Autodesk Inventor part; units mm, degrees
ref_plane "YZ Plane" through (0, 0, 0) normal (1, 0, 0) x (0, 1, 0)
ref_plane "XZ Plane" through (0, 0, 0) normal (0, 1, 0) x (-1, 0, 0)
ref_plane "XY Plane" through (0, 0, 0) normal (0, 0, 1) x (1, 0, 0)
sketch "Эскиз1" plane through (0, 0, 0) normal (0, 1, 0) x (-1, 0, 0)
  arc A0 (42, 49.6085) -> (42, -49.6085) centre (0, 0) ccw
  line L0 (42, 49.6085) -> (42, -49.6085)
  arc A1 (42, -49.6085) -> (42, 49.6085) centre (0, 0) ccw construction
  line L1 (34, 55.3986) -> (34, -55.3986) construction
  circle A2 centre (34, 45) radius 1.5
  circle A3 centre (34, -45) radius 1.5
  line L2 (-28, 58.66) -> (-28, -58.66) construction
  line L3 (0, 0) -> (-28, -55) construction
  line L4 (0, 0) -> (-56.516, 0) construction
  circle A4 centre (-56.516, 0) radius 2
  circle A5 centre (-28, 45) radius 1.5
  circle A6 centre (-28, -45) radius 1.5
  dimension "d0" = 130
  dimension "d1" = 42
  dimension "d4" = 8
  dimension "d5" = 3
  dimension "d6" = 3
  dimension "d7" = 45
  dimension "d8" = 45
  dimension "d9" = 70
  dimension "d12" = 55
  dimension "d16" = 61.7171
  dimension "d18" = 4
  dimension "d20" = 3
  dimension "d21" = 45
  dimension "d22" = 3
  dimension "d38" = 56.516
extrude "Выдавливание1" add sketch "Эскиз1" along normal blind 3
sketch "Эскиз2" plane through (0, 3, 0) normal (0, 1, 0) x (1, 0, 0)
  circle A0 centre (-34, -45) radius 1.5
  circle A1 centre (-34, 45) radius 1.5
  line L0 (-34, -45) -> (-34, 45) construction
  circle A2 centre (0, 0) radius 55 construction
  line L1 (0, 0) -> (0, -55) construction
  line L2 (0, 0) -> (45.0534, -31.5467) construction
  circle A3 centre (45.0534, -31.5467) radius 1.5
  circle A4 centre (56.516, 0) radius 2
  line L3 (0, 0) -> (56.516, 0) construction
  circle A5 centre (45.0534, 31.5467) radius 1.5
  circle A6 centre (-34, -32) radius 1.5
  circle A7 centre (-34, 32) radius 1.5
  line L4 (-42, 49.6085) -> (-42, -49.6085)
  point P0 (-42, 0)
  point P1 (-34, 0)
  dimension "d25" = 110
  dimension "d26" = 55
  dimension "d28" = 3
  dimension "d34" = 3
  dimension "d35" = 3
  dimension "d36" = 32
  dimension "d37" = 32
extrude "Выдавливание2" cut sketch "Эскиз2" against normal blind 10 contours A3 | A5 | A6 | A7
chamfer "Фаска1" distance 1.6 angle 45 4 edges at (43.5534, 0, 31.5467) (43.5534, 0, -31.5467) (-35.5, 0, -32) (-35.5, 0, 32)
sketch "Эскиз3" plane through (0, 3, 0) normal (0, 1, 0) x (1, 0, 0)
  circle A0 centre (-34, -45) radius 1.5
  circle A1 centre (-34, 45) radius 1.5
  line L0 (-34, -45) -> (-34, 45) construction
  line L1 (-34, 45) -> (12.5, 45) construction
  line L2 (-10.75, 45) -> (-10.75, -55.9117) construction
  circle A2 centre (-10.75, -30) radius 1.5
  circle A3 centre (-10.75, 30) radius 1.5
  point P0 (0, 0)
  dimension "d39" = 46.5
  dimension "d40" = 3
  dimension "d41" = 3
  dimension "d42" = 30
  dimension "d43" = 30
extrude "Выдавливание3" cut sketch "Эскиз3" against normal blind 10 contours A2 | A3
sketch "Эскиз4" plane through (0, 3, 0) normal (0, 1, 0) x (1, 0, 0)
  arc A0 (42.2049, -65) -> (42.2049, 65) centre (0, 0) ccw
  arc A1 (-42, -49.6085) -> (-42, 49.6085) centre (0, 0) ccw
  line L0 (0, -65) -> (42.2049, -65)
  line L1 (0, 65) -> (42.2049, 65)
  arc A2 (42.2049, 65) -> (42.2049, -65) centre (0, 0) ccw construction
  line L2 (0, 0) -> (65, 0) construction
  line L3 (0, 0) -> (75.9442, -15.451) construction
  line L4 (0, 0) -> (70.522, -32.1387) construction
  line L5 (0, 0) -> (54.3205, -55.2769) construction
  line L6 (0, 0) -> (57.5937, 51.8576) construction
  line L7 (0, 0) -> (41.0687, 65.7237) construction
  circle A3 centre (0, 0) radius 70.5 construction
  arc A4 (43.3889, -55.5666) -> (54.8009, -44.3521) centre (0, 0) ccw construction
  arc A5 (44.9275, -57.5371) -> (56.7442, -45.9249) centre (0, 0) ccw
  arc A6 (41.8503, -53.5962) -> (52.8576, -42.7793) centre (0, 0) ccw
  arc A7 (41.8503, -53.5962) -> (44.9275, -57.5371) centre (43.3889, -55.5666) ccw
  arc A8 (56.7442, -45.9249) -> (52.8576, -42.7793) centre (54.8009, -44.3521) ccw
  arc A9 (62.8501, -31.9393) -> (65.3382, -26.4795) centre (0, 0) ccw construction
  arc A10 (65.0788, -33.0719) -> (67.6552, -27.4185) centre (0, 0) ccw
  arc A11 (60.6214, -30.8067) -> (63.0213, -25.5405) centre (0, 0) ccw
  arc A12 (60.6214, -30.8067) -> (65.0788, -33.0719) centre (62.8501, -31.9393) ccw
  arc A13 (67.6552, -27.4185) -> (63.0213, -25.5405) centre (65.3382, -26.4795) ccw
  arc A14 (68.424, -16.9825) -> (69.6202, -11.1029) centre (0, 0) ccw construction
  arc A15 (70.8504, -17.5847) -> (72.089, -11.4967) centre (0, 0) ccw
  arc A16 (65.9976, -16.3803) -> (67.1514, -10.7092) centre (0, 0) ccw
  arc A17 (65.9976, -16.3803) -> (70.8504, -17.5847) centre (68.424, -16.9825) ccw
  arc A18 (72.089, -11.4967) -> (67.1514, -10.7092) centre (69.6202, -11.1029) ccw
  arc A19 (57.4063, 40.9238) -> (39.8696, 58.1435) centre (0, 0) ccw construction
  arc A20 (59.442, 42.375) -> (41.2834, 60.2053) centre (0, 0) ccw
  arc A21 (55.3707, 39.4726) -> (38.4558, 56.0817) centre (0, 0) ccw
  arc A22 (55.3707, 39.4726) -> (59.442, 42.375) centre (57.4063, 40.9238) ccw
  arc A23 (41.2834, 60.2053) -> (38.4558, 56.0817) centre (39.8696, 58.1435) ccw
  line L8 (0, 0) -> (75.9442, 15.451) construction
  line L9 (0, 0) -> (70.522, 32.1387) construction
  arc A24 (65.3382, 26.4795) -> (62.8501, 31.9393) centre (0, 0) ccw construction
  arc A25 (67.6552, 27.4185) -> (65.0788, 33.0719) centre (0, 0) ccw
  arc A26 (63.0213, 25.5405) -> (60.6214, 30.8067) centre (0, 0) ccw
  arc A27 (65.0788, 33.0719) -> (60.6214, 30.8067) centre (62.8501, 31.9393) ccw
  arc A28 (63.0213, 25.5405) -> (67.6552, 27.4185) centre (65.3382, 26.4795) ccw
  arc A29 (69.6202, 11.1029) -> (68.424, 16.9825) centre (0, 0) ccw construction
  arc A30 (72.089, 11.4967) -> (70.8504, 17.5847) centre (0, 0) ccw
  arc A31 (67.1514, 10.7092) -> (65.9976, 16.3803) centre (0, 0) ccw
  arc A32 (70.8504, 17.5847) -> (65.9976, 16.3803) centre (68.424, 16.9825) ccw
  arc A33 (67.1514, 10.7092) -> (72.089, 11.4967) centre (69.6202, 11.1029) ccw
  point P0 (21.1024, -65)
  dimension "d46" = 155
  dimension "d53" = 11.5
  dimension "d54" = 24.5
  dimension "d55" = 45.5
  dimension "d56" = 42
  dimension "d57" = 58
  dimension "d58" = 65
  dimension "d60" = 65
  dimension "d61" = 141
  dimension "d62" = 5
  dimension "d63" = 5
  dimension "d64" = 5
  dimension "d65" = 8
  dimension "d66" = 3
  dimension "d67" = 3
  dimension "d68" = 3
  dimension "d69" = 3
  dimension "d70" = 2.5
  dimension "d71" = 8
  dimension "d72" = 8
  dimension "d73" = 3
extrude "Выдавливание4" add sketch "Эскиз4" against normal blind 3
fillet "Сопряжение2" radius 15 2 edges at (42.2049, 1.5, 65) (42.2049, 1.5, -65)
sketch "Эскиз5" plane through (0, 3, 0) normal (0, 1, 0) x (1, 0, 0)
  line L0 (24, -72) -> (24, 72) construction
  arc A0 (41.8503, -53.5962) -> (52.8576, -42.7793) centre (0, 0) ccw
  arc A1 (56.7442, -45.9249) -> (52.8576, -42.7793) centre (54.8009, -44.3521) ccw
  arc A2 (44.9275, -57.5371) -> (56.7442, -45.9249) centre (0, 0) ccw
  arc A3 (41.8503, -53.5962) -> (44.9275, -57.5371) centre (43.3889, -55.5666) ccw
  arc A4 (60.6214, -30.8067) -> (63.0213, -25.5405) centre (0, 0) ccw
  arc A5 (67.6552, -27.4185) -> (63.0213, -25.5405) centre (65.3382, -26.4795) ccw
  arc A6 (65.0788, -33.0719) -> (67.6552, -27.4185) centre (0, 0) ccw
  arc A7 (60.6214, -30.8067) -> (65.0788, -33.0719) centre (62.8501, -31.9393) ccw
  arc A8 (65.9976, -16.3803) -> (67.1514, -10.7092) centre (0, 0) ccw
  arc A9 (72.089, -11.4967) -> (67.1514, -10.7092) centre (69.6202, -11.1029) ccw
  arc A10 (70.8504, -17.5847) -> (72.089, -11.4967) centre (0, 0) ccw
  arc A11 (65.9976, -16.3803) -> (70.8504, -17.5847) centre (68.424, -16.9825) ccw
  arc A12 (55.3707, 39.4726) -> (38.4558, 56.0817) centre (0, 0) ccw
  arc A13 (41.2834, 60.2053) -> (38.4558, 56.0817) centre (39.8696, 58.1435) ccw
  arc A14 (59.442, 42.375) -> (41.2834, 60.2053) centre (0, 0) ccw
  arc A15 (55.3707, 39.4726) -> (59.442, 42.375) centre (57.4063, 40.9238) ccw
  arc A16 (67.1514, 10.7092) -> (65.9976, 16.3803) centre (0, 0) ccw
  arc A17 (70.8504, 17.5847) -> (65.9976, 16.3803) centre (68.424, 16.9825) ccw
  arc A18 (72.089, 11.4967) -> (70.8504, 17.5847) centre (0, 0) ccw
  arc A19 (67.1514, 10.7092) -> (72.089, 11.4967) centre (69.6202, 11.1029) ccw
  arc A20 (63.0213, 25.5405) -> (67.6552, 27.4185) centre (65.3382, 26.4795) ccw
  arc A21 (63.0213, 25.5405) -> (60.6214, 30.8067) centre (0, 0) ccw
  arc A22 (65.0788, 33.0719) -> (60.6214, 30.8067) centre (62.8501, 31.9393) ccw
  arc A23 (67.6552, 27.4185) -> (65.0788, 33.0719) centre (0, 0) ccw
  circle A24 centre (-10.75, 30) radius 1.5
  circle A25 centre (-10.75, -30) radius 1.5
  circle A26 centre (45.0534, 31.5467) radius 1.5
  circle A27 centre (-34, 32) radius 1.5
  circle A28 centre (45.0534, -31.5467) radius 1.5
  circle A29 centre (-34, -32) radius 1.5
  arc A30 (46.5, 62) -> (37.5, 65) centre (37.5, 50) ccw
  line L1 (37.5, 65) -> (0, 65)
  arc A31 (0, 65) -> (-42, 49.6085) centre (0, 0) ccw
  line L2 (-42, 49.6085) -> (-42, -49.6085)
  arc A32 (-42, -49.6085) -> (0, -65) centre (0, 0) ccw
  line L3 (0, -65) -> (37.5, -65)
  arc A33 (37.5, -65) -> (46.5, -62) centre (37.5, -50) ccw
  arc A34 (46.5, -62) -> (46.5, 62) centre (0, 0) ccw
  circle A35 centre (28, 45) radius 1.5
  circle A36 centre (28, -45) radius 1.5
  circle A37 centre (56.516, 0) radius 2
  circle A38 centre (-34, 45) radius 1.5
  circle A39 centre (-34, -45) radius 1.5
  arc A40 (46.5, -62) -> (46.5, 62) centre (0, 0) ccw
  arc A41 (-42, -49.6085) -> (0, -65) centre (0, 0) ccw
  circle A42 centre (24, -72) radius 10.5
  circle A43 centre (24, 72) radius 10.5
  dimension "d74" = 72
  dimension "d75" = 72
  dimension "d76" = 32.516
  dimension "d77" = 21
  dimension "d78" = 21
extrude "Выдавливание5" cut sketch "Эскиз5" against normal blind 3 contours A43 L1 | L1 A43 | A42 L3 | L3 A42
fillet "Сопряжение3" radius 8 4 edges at (31.8262, 1.5, 65) (16.1738, 1.5, 65) (16.1738, 1.5, -65) (31.8262, 1.5, -65)
equation "\"d60\" = d58"
equation "\"d67\" = d66"
properties part number "V_3"
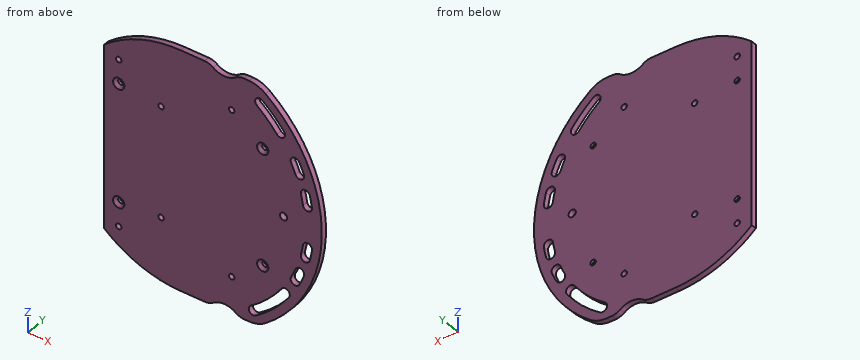
Read the model definition and answer for the solid it produces. Units are mm, in the model's axes. Round coordinates to 2 decimals unless told otherwise and drop trailing zeros. Write each loop counter-clockwise with the first axis right and the second up, starting at its lowest first coordinate (ties: lowest second). Pieces come first, ordered by that corner, then holes. Notation, with made-up numbers: (-20.75, 57.25) - (13.25, 57.25) arc R25 ccw to (13.25, 93.25) - close; hole circle Ø8 at (21, -31.75). An arc over 180 degrees is marked (long way). One line per item, written item: value.
Q1. Find section B-B (x = -34). Determine the outline of the cut face in (y, z).
The answers:
outline: (0, -55.4) - (3, -55.4) - (3, -46.5) - (0, -46.5) - close; (0, -43.5) - (3, -43.5) - (3, -33.5) - (1.6, -33.5) - (0, -35.1) - close; (0, -28.9) - (1.6, -30.5) - (3, -30.5) - (3, 30.5) - (1.6, 30.5) - (0, 28.9) - close; (0, 35.1) - (1.6, 33.5) - (3, 33.5) - (3, 43.5) - (0, 43.5) - close; (0, 46.5) - (3, 46.5) - (3, 55.4) - (0, 55.4) - close
Q2. This flat-tipped pin is pushed along its axis until it touches: P1, Ø5, axis at x = -34, z = -32, coming from the -Y side. Where does it stop, or does it pass through?
The answers:
P1: stops at y = 0.6
Q3. Find section A-A (z = 0). Determine the outline of the cut face in (x, y), and give its area (4 significant figures).
The answers:
outline: (-42, 0) - (54.52, 0) - (54.52, 3) - (-42, 3) - close; (58.52, 0) - (77.5, 0) - (77.5, 3) - (58.52, 3) - close
area: 346.5 mm2
Q4. Find section D-D (z = -45). Determine the outline of the cut face in (x, y), and give its area (3 significant figures).
The answers:
outline: (-42, 0) - (-35.5, 0) - (-35.5, 3) - (-42, 3) - close; (-32.5, 0) - (26.5, 0) - (26.5, 3) - (-32.5, 3) - close; (29.5, 0) - (50.98, 0) - (50.98, 3) - (29.5, 3) - close; (57.48, 0) - (63.1, 0) - (63.1, 3) - (57.48, 3) - close
area: 278 mm2
Q5. Find section C-C (x = -10.75). Determine the outline of the cut face in (y, z).
The answers:
outline: (0, -64.1) - (3, -64.1) - (3, -31.5) - (0, -31.5) - close; (0, -28.5) - (3, -28.5) - (3, 28.5) - (0, 28.5) - close; (0, 31.5) - (3, 31.5) - (3, 64.1) - (0, 64.1) - close
Q6. Straight lines are drawn through the part: line 1 (Z direction, x = -34, y = 2.05); line 2 (Z direction, x = 70.5, y = 2.3); line 3 (Z direction, x = 55, y = 1.9). For each, find the intervals that lie inside material, in ascending order. Write a range as from..to.
The answers:
line 1: z = -55.4..-46.5, -43.5..-33.5, -30.5..30.5, 33.5..43.5, 46.5..55.4
line 2: z = -32.19..-18.38, -8.76..8.76, 18.38..32.19
line 3: z = -54.6..-48, -39.99..-1.3, 1.3..41.86, 48..54.6
